Source: CAD feature listing. Evaluate the final solid. Frame: model axes, mm. A direction names the side the tool comes from. Give positions to 0.01 mm unless a question says otherwise; leave off trailing zeros. Write each loop counter-clockwise with the first axis right and the second up, starting at its lowest first coordinate (ties: lowest second). Pieces come first, ordered by that corner, then holes. Notation, with made-up numbers: (71, 55.25) -> (79, 55.25) arc R24 ccw to (79, 71.25) -> close; hole circle Ø8 at (46, 0.25). An arc over 180 degrees is marked (long way). Answer as a JSON object with one key per item and string values. Group by question number.
Item 1: First-contact query: pin 1 Ø11 at (x, z) = (-57.5, 17) entering from -Y. Flat tip, straight axial feed; report the tip coordinate or a pass-through.
Item 2: Pull-direction query (X, two-part tool) for faces 1 (the face through (60.547, 17.339, 16.866)), 2 (the face through (-1, 14, 32)); classes: pulls with the +X half, pulls with the -X half, needs draft (parallel to the pull), parting line crosses it, or undercut.
Item 3: Section query A-A on z = -13. Return the cut outline in (x, y).
Item 4: Section query D-D on z = -23.5. Return the cut outline in (x, y), plus the area to 3 significant figures.
Item 5: Ray query, probe 1 along Z at (x, y) = (36.5, 10); probe 2 along X at (y, z) = (7.75, 22); probe 3 along Z at (x, y) = (57.5, 3.6). Return the intervals inside material, ascending. Write a range as from..to.
Item 6: Section query B-B on x = 36.5. Return the cut outline in (y, z), plus the area to 3 significant figures.
Item 7: Access query for faces 3 (the face through (51.506, 2.958, -12.736)), 4 (the face through (37.77, 14.7, -25.07)). Directions: +Z, -Z, +X, -X, +Y, -Y. A direction counts if a zero-diameter tool reaches every point of the face in a straight line with its end or side. Return the directions, or none.
Item 8: Section query C-C on y = 25.25. Give the number of separate pieces and of enclosed holes in the cut face, plus the area to 3 significant figures.
Autodesk Inventor part; units mm, degrees
ref_plane "YZ Plane" through (0, 0, 0) normal (1, 0, 0) x (0, 1, 0)
ref_plane "XZ Plane" through (0, 0, 0) normal (0, 1, 0) x (-1, 0, 0)
ref_plane "XY Plane" through (0, 0, 0) normal (0, 0, 1) x (1, 0, 0)
sketch "Sketch1" plane through (0, 0, 0) normal (0, 1, 0) x (-1, 0, 0)
  line L0 (72.5, 32) -> (-72.5, 32)
  line L1 (-72.5, 32) -> (-72.5, -32)
  line L2 (-72.5, -32) -> (72.5, -32)
  line L3 (72.5, -32) -> (72.5, 32)
  line L4 (72.5, 32) -> (-72.5, -32) construction
  line L5 (-72.5, 32) -> (72.5, -32) construction
  line L6 (0, 0) -> (0, -32) construction
  line L7 (0, 0) -> (0, 32) construction
  circle A0 centre (0, -13) radius 3.05
  circle A1 centre (0, 16) radius 3.05
  circle A2 centre (57.5, -13) radius 3.05
  circle A3 centre (57.5, 17) radius 3.05
  line L8 (57.5, -13) -> (57.5, 17) construction
  circle A4 centre (-57.5, -13) radius 3.05
  circle A5 centre (-57.5, 17) radius 3.05
  point P0 (57.5, 2)
  dimension "d0" = 145
  dimension "d1" = 64
  dimension "d2" = 6.1
  dimension "d3" = 6.1
  dimension "d4" = 15
  dimension "d5" = 30
  dimension "d18" = 2
extrude "Extrusion1" add sketch "Sketch1" along normal blind 29
sketch "Sketch2" plane through (0, 0, 0) normal (0, -1, 0) x (1, 0, 0)
  arc A0 (-35.5, 17.5) -> (-35.5, 26.5) centre (-35.5, 22) ccw
  line L0 (-37.5, 17.5) -> (-35.5, 17.5)
  arc A1 (-37.5, 26.5) -> (-37.5, 17.5) centre (-37.5, 22) ccw
  line L1 (-35.5, 26.5) -> (-37.5, 26.5)
  line L2 (-35.5, -17.5) -> (-37.5, -17.5)
  arc A2 (-35.5, -26.5) -> (-35.5, -17.5) centre (-35.5, -22) ccw
  line L3 (-37.5, -26.5) -> (-35.5, -26.5)
  arc A3 (-37.5, -17.5) -> (-37.5, -26.5) centre (-37.5, -22) ccw
  line L4 (35.5, -26.5) -> (37.5, -26.5)
  arc A4 (35.5, -17.5) -> (35.5, -26.5) centre (35.5, -22) ccw
  line L5 (37.5, -17.5) -> (35.5, -17.5)
  arc A5 (37.5, -26.5) -> (37.5, -17.5) centre (37.5, -22) ccw
  line L6 (37.5, 26.5) -> (35.5, 26.5)
  arc A6 (37.5, 17.5) -> (37.5, 26.5) centre (37.5, 22) ccw
  line L7 (35.5, 17.5) -> (37.5, 17.5)
  arc A7 (35.5, 26.5) -> (35.5, 17.5) centre (35.5, 22) ccw
  circle A8 centre (36.5, 0) radius 4.5
  circle A9 centre (-36.5, 0) radius 4.5
  line L8 (47, -32) -> (-47, -32)
  line L9 (47, 32) -> (47, -32)
  line L10 (-47, 32) -> (47, 32)
  line L11 (-47, -32) -> (-47, 32)
  circle A10 centre (0, 0) radius 20
  line L12 (-37.5, -22) -> (-35.5, -22)
  line L13 (35.5, -22) -> (37.5, -22)
  line L14 (35.5, 22) -> (37.5, 22)
  line L15 (-37.5, 22) -> (-35.5, 22)
  point P0 (0, 0)
  point P1 (-36.5, -22)
  point P2 (-36.5, 22)
  point P3 (36.5, 22)
  point P4 (36.5, -22)
hole "Hole1" at (-36.5, 0, -22) at (-36.5, 0, 22) at (36.5, 0, 22) at (36.5, 0, -22) direction (0, 1, 0) diameter 6.647 end through all
sketch "Sketch4" plane through (0, 0, 0) normal (0, -1, 0) x (1, 0, 0)
  circle A0 centre (-57.5, 17) radius 3.05
  circle A1 centre (-57.5, -13) radius 3.05
  circle A2 centre (0, -13) radius 3.05
  circle A3 centre (0, 16) radius 3.05
  circle A4 centre (57.5, 17) radius 3.05
  circle A5 centre (57.5, -13) radius 3.05
  circle A6 centre (-57.5, 17) radius 6
  circle A7 centre (-57.5, -13) radius 6
  circle A8 centre (0, 16) radius 6
  circle A9 centre (0, -13) radius 6
  circle A10 centre (57.5, 17) radius 6
  circle A11 centre (57.5, -13) radius 6
  point P0 (0, 0)
  dimension "d15" = 12
extrude "Extrusion2" cut sketch "Sketch4" against normal blind 6 contours A0 | A1 | A2 | A3 | A4 | A5 | A6 | A7 | A8 | A9 | A10 | A11
properties part number "assist_wheel_bracket"
Worked answers:
{
 "1": {"pin 1": "y = 6"},
 "2": {"face 1": "undercut", "face 2": "needs draft"},
 "3": {"outline": "(-72.5, 0) -> (-63.5, 0) -> (-63.5, 6) -> (-60.55, 6) -> (-60.55, 29) -> (-72.5, 29) -> close; (-54.45, 6) -> (-51.5, 6) -> (-51.5, 0) -> (-6, 0) -> (-6, 6) -> (-3.05, 6) -> (-3.05, 29) -> (-54.45, 29) -> close; (3.05, 6) -> (6, 6) -> (6, 0) -> (51.5, 0) -> (51.5, 6) -> (54.45, 6) -> (54.45, 29) -> (3.05, 29) -> close; (60.55, 6) -> (63.5, 6) -> (63.5, 0) -> (72.5, 0) -> (72.5, 29) -> (60.55, 29) -> close"},
 "4": {"outline": "(-72.5, 0) -> (-39.47, 0) -> (-39.47, 29) -> (-72.5, 29) -> close; (-33.53, 0) -> (33.53, 0) -> (33.53, 29) -> (-33.53, 29) -> close; (39.47, 0) -> (72.5, 0) -> (72.5, 29) -> (39.47, 29) -> close", "area": "3,860 mm^2"},
 "5": {"probe 1": "-32..-25.32, -18.68..18.68, 25.32..32", "probe 2": "-72.5..-39.82, -33.18..33.18, 39.82..72.5", "probe 3": "-32..-19, -7..11, 23..32"},
 "6": {"outline": "(0, -32) -> (29, -32) -> (29, -25.32) -> (0, -25.32) -> close; (0, -18.68) -> (29, -18.68) -> (29, 18.68) -> (0, 18.68) -> close; (0, 25.32) -> (29, 25.32) -> (29, 32) -> (0, 32) -> close", "area": "1,470 mm^2"},
 "7": {"face 3": "-Y", "face 4": "+Y, -Y"},
 "8": {"separate pieces": "1", "enclosed holes": "10", "area": "8,970 mm^2"}
}
